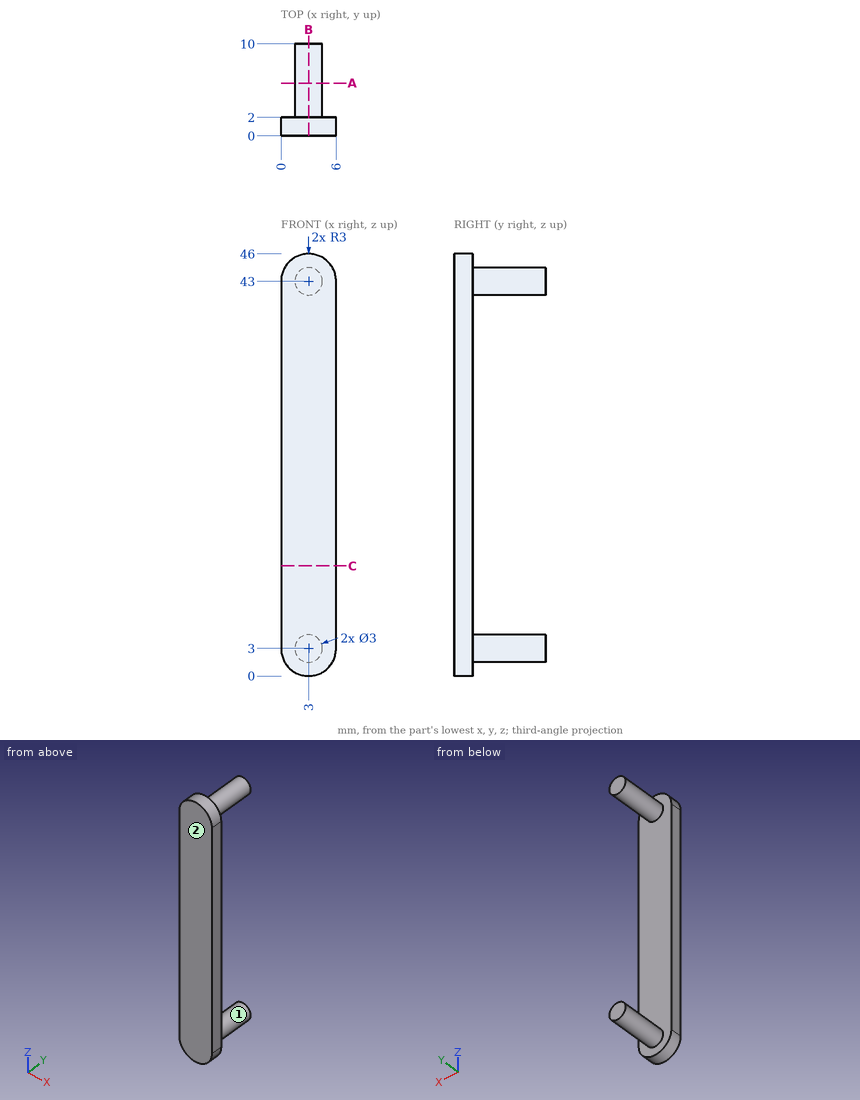
Answer from the drawing. Dimensions are ordinates in mm from the lowest x, y and z of the part. A direction names the side the tool comes from. Round coordinates to 2 decimals unless told otherwise and drop trailing zeros. Write each loop counter-clockwise with the first axis right and the second up, starting at its lowest first coordinate (ties: lowest second). Pieces come first, ordered by that corner, then holes. Notation, with made-up numbers: (63, 84) -> (67, 84) arc R28 cw to (67, 114) -> close; hole circle Ø1 at (42, 63). An arc over 180 degrees is marked (long way). Answer in a Markdown table with one row per item. Add a question column.
1) Find section C-C, the plane z = 12. Determine the outline of the cut face in (x, y).
2) Find section B-B, the plane x = 3. Determine the outline of the cut face in (y, z).
3) Consider line 1 (Y direction, x = 3.9, z = 27); line 2 (Z direction, x = 2.2, y = 5.75); line 3 (Z direction, x = 2.55, y = 7). Determine where each line is inside the solid, lowest interval first.
4) Find section A-A, the plane y = 5.75. Determine the outline of the cut face in (x, z), and give its area (3 significant figures).
5) Which of the six approach directions +Z, -Z, +X, -X, +Y, -Y give full straight-line access (tool end or side, diameter ignored) to the marked faces 1 and 2?
6) Given P1, Ø3, axis at x = 3.5, z = 11.5, coming from the +Y side, flat-ended and moving along its own axis, determine where the tip first touches the part or whether it passes through.
Findings below:
| question | item | result |
|---|---|---|
| 1 | outline | (0, 0) -> (6, 0) -> (6, 2) -> (0, 2) -> close |
| 2 | outline | (0, 0) -> (2, 0) -> (2, 1.5) -> (10, 1.5) -> (10, 4.5) -> (2, 4.5) -> (2, 41.5) -> (10, 41.5) -> (10, 44.5) -> (2, 44.5) -> (2, 46) -> (0, 46) -> close |
| 3 | line 1 | 0 to 2 |
| 3 | line 2 | 1.73 to 4.27, 41.73 to 44.27 |
| 3 | line 3 | 1.57 to 4.43, 41.57 to 44.43 |
| 4 | outline | circle Ø3 at (3, 3); circle Ø3 at (3, 43) |
| 4 | area | 14.1 mm² |
| 5 | face 1 | +Y |
| 5 | face 2 | +Z, -Z, +X, -X, -Y |
| 6 | P1 | y = 2 |
